Work out the finished part from the listing and answer in its coordinate system (mm). A direction names the side the tool comes from. Round coordinates to 2 decimals unless told otherwise and drop trailing zeros. One line per item, written item: value.
```python
from build123d import *

# Parameters (mm, degrees)
BOSS_EXTRUDE1_DEPTH = 1000
SKETCH2_R           = 2
CUT_EXTRUDE1_DEPTH  = 1000


with BuildPart() as part:
    # Sketch1 → Boss-Extrude1 (new body)
    with BuildSketch(Plane.XY):
        with BuildLine():
            Line((-100, 0), (-100, 2))
            Line((-100, 2), (-80, 2))
            add(Edge.make_bspline(
                [(-80, 2), (-43.592140665, 8.040624859), (9.738592922, -1.468299524), (63.334289404, 7.534924383), (80, 2)],
                knots=[0, 0, 0, 0, 0.681210574, 1, 1, 1, 1], degree=3))
            Line((80, 2), (102, 2))
            Line((102, 2), (102, 0))
            Line((102, 0), (80, 0))
            add(Edge.make_bspline(
                [(-80, 0), (-43.571889954, 5.402355935), (9.739082816, -3.252830544), (63.415202278, 6.17713334), (80, 0)],
                knots=[0, 0, 0, 0, 0.680838855, 1, 1, 1, 1], degree=3))
            Line((-80, 0), (-100, 0))
        make_face()
    extrude(amount=-BOSS_EXTRUDE1_DEPTH)

    # Sketch2 → Cut-Extrude1 (cut)
    with BuildSketch(Plane(origin=(0, 2, 0), x_dir=(1, 0, 0), z_dir=(0, 1, 0))):
        with Locations(Location((91, 950, 0), (0, 0, 180))):
            Circle(SKETCH2_R)
        with Locations(Location((-90, 950, 0), (0, 0, 180))):
            Circle(SKETCH2_R)
        with Locations(Location((91, 850, 0), (0, 0, 180))):
            Circle(SKETCH2_R)
        with Locations(Location((-90, 850, 0), (0, 0, 180))):
            Circle(SKETCH2_R)
        with Locations(Location((91, 750, 0), (0, 0, 180))):
            Circle(SKETCH2_R)
        with Locations(Location((-90, 750, 0), (0, 0, 180))):
            Circle(SKETCH2_R)
        with Locations(Location((91, 650, 0), (0, 0, 180))):
            Circle(SKETCH2_R)
        with Locations(Location((-90, 650, 0), (0, 0, 180))):
            Circle(SKETCH2_R)
        with Locations(Location((91, 550, 0), (0, 0, 180))):
            Circle(SKETCH2_R)
        with Locations(Location((-90, 550, 0), (0, 0, 180))):
            Circle(SKETCH2_R)
        with Locations(Location((91, 450, 0), (0, 0, 180))):
            Circle(SKETCH2_R)
        with Locations(Location((-90, 450, 0), (0, 0, 180))):
            Circle(SKETCH2_R)
        with Locations(Location((91, 350, 0), (0, 0, 180))):
            Circle(SKETCH2_R)
        with Locations(Location((-90, 350, 0), (0, 0, 180))):
            Circle(SKETCH2_R)
        with Locations(Location((91, 250, 0), (0, 0, 180))):
            Circle(SKETCH2_R)
        with Locations(Location((-90, 250, 0), (0, 0, 180))):
            Circle(SKETCH2_R)
        with Locations(Location((91, 150, 0), (0, 0, 180))):
            Circle(SKETCH2_R)
        with Locations(Location((-90, 150, 0), (0, 0, 180))):
            Circle(SKETCH2_R)
        with Locations(Location((91, 50, 0), (0, 0, 180))):
            Circle(SKETCH2_R)
        with Locations(Location((-90, 50, 0), (0, 0, 180))):
            Circle(SKETCH2_R)
    extrude(amount=-CUT_EXTRUDE1_DEPTH, mode=Mode.SUBTRACT)


solid = part.part
```
1) Each of these flat-tipped pins is pushed along its axis until it touches: pin 1 (2 mm diameter, centred on x = -24.5, y = 1.5, fed in from -Z); pin 2 (2.5 mm diameter, centred on x = 91, z = -250, fed in from +Y); pin 3 (6.5 mm diameter, centred on x = -90, z = -450, fed in from +Y). Where does it stop, or does it pass through?
Check values:
pin 1: z = -1000
pin 2: through
pin 3: y = 2
2) Find the intervals of material crossed by probe 1 along Y at (x, z) = (31.5, -382); probe 2 along Y at (x, z) = (93, -951.5), in increasing order. Write a range as from..to.
Check values:
probe 1: 2.17..3.82
probe 2: 0..2
3) For faces 1 (the face through (-90, 0, -493)), 2 (the face through (-90, 2, -493)), 3 (the face through (91, 2, -493)), determine the directions among +Z, -Z, +X, -X, +Y, -Y from which every point of the face is accessible in a straight line to the end or side of a thin tool.
Check values:
face 1: +Z, -Z, +X, -X, -Y
face 2: +Z, -Z, -X, +Y
face 3: +Z, -Z, +X, +Y
